from build123d import *

# Parameters (mm, degrees)
F0_W     = 63.351966
F0_H     = 58.721166
F1_DEPTH = 50.8
F2_R     = 6.67715
F3_DEPTH = 25.4
F4_R     = 5.78901
F5_DEPTH = 25.4
F6_R     = 13.653807
F7_DEPTH = 38.1


with BuildPart() as f1:
    # F0 (on Top) → F1 (new body)
    with BuildSketch(Plane.XY):
        with Locations((31.675983, 29.360583)):
            Rectangle(F0_W, F0_H)
    extrude(amount=F1_DEPTH)

    # F2 (on face) → F3 (cut)
    with BuildSketch(Plane.XY.offset(50.8)):
        with Locations((47.149416, 48.132766)):
            Circle(F2_R)
    extrude(amount=-F3_DEPTH, mode=Mode.SUBTRACT)

    # F4 (on face) → F5 (cut)
    with BuildSketch(Plane(origin=(0, 0, 0), x_dir=(1, 0, 0), z_dir=(0, 0, -1))):
        with Locations((9.225111, -8.943532)):
            Circle(F4_R)
    extrude(amount=-F5_DEPTH, mode=Mode.SUBTRACT)

    # F6 (on face) → F7 (cut)
    with BuildSketch(Plane(origin=(0, 0, 0), x_dir=(0, -1, 0), z_dir=(-1, 0, 0))):
        with Locations((0, 50.8)):
            Circle(F6_R)
    extrude(amount=-F7_DEPTH, mode=Mode.SUBTRACT)


solid = f1.part
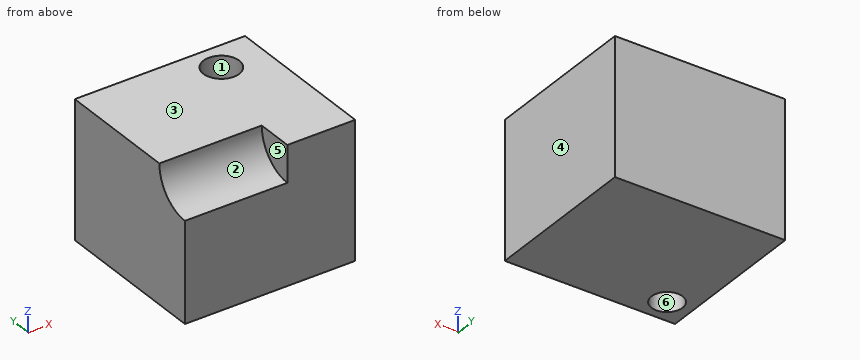
Verification items for the finished model (mm, model axes). Face numbers are marked on the shaded views. A direction names the side the tool comes from. Coordinates: 2 decimals unless noted, no trailing zeros. Order: outer loops, then holes, each group sorted by start corner. A loop starts at its lowest first (then second) coordinate and runs counter-clockwise, first axis right, second up. Notation, with made-up numbers: (13.25, -2) -> (18.25, -2) arc R17 cw to (18.25, 11) -> close; hole circle Ø9 at (66.25, 66). An arc over 180 degrees is marked (long way). Put each result on its own line as item: value. Start each with the question number.
1. Access from +Z, -Z, +X, -X, +Y, -Y to the whole of each face (thin tool, end or side, straight path). Record for the marked faces 4, 5 and 6.
2. Cross-section at B-B, the plane y = 49.5. Record the boundary of the cut face in (x, z), then the cut area to 3 significant figures.
3. Cross-section at D-D, the plane x = 25. Record the boundary of the cut face in (y, z), then the cut area to 3 significant figures.
4. Cross-section at A-A, the plane x = 8. Record the boundary of the cut face in (y, z), then the cut area to 3 significant figures.
5. Material ranges on L1, parallel to X at y = 8.5, z = 21.5; L2, parallel to Z at x = 50, y = 42.5; L3, parallel to Y at x = 49, z = 40.5, recorded low to high. Write a range as [from, to].
6. Go/stop test with flat-tipped pins: pin 1 Ø7 at (y, z) = (4.5, 45) entering from -X; pin 2 Ø10.5 at (x, y) = (47.15, 48.13) entering from +Z. Record where each tip stops, or that it passes through.
7. Mould release check, pull along Y, two halves, no side actions. Record for the marked faces 1, 2 and 3: released by +Y, released by -Y, zero draft, split by the parting line, or undercut.
8. Cross-section at C-C, the plane z = 13.5. Record the boundary of the cut face in (x, y).
Computed:
1. face 4: +Z, -Z, +X, +Y, -Y
1. face 5: +Z, -X, -Y
1. face 6: -Z
2. outline: (0, 0) -> (63.35, 0) -> (63.35, 50.8) -> (53.69, 50.8) -> (53.69, 25.4) -> (40.61, 25.4) -> (40.61, 50.8) -> (0, 50.8) -> close
2. area: 2,890 mm2
3. outline: (0, 0) -> (58.72, 0) -> (58.72, 50.8) -> (13.65, 50.8) arc R13.65 cw to (0, 37.15) -> close
3. area: 2,840 mm2
4. outline: (0, 0) -> (3.29, 0) -> (3.29, 25.4) -> (14.6, 25.4) -> (14.6, 0) -> (58.72, 0) -> (58.72, 50.8) -> (13.65, 50.8) arc R13.65 cw to (0, 37.15) -> close
4. area: 2,550 mm2
5. L1: [0, 3.45], [15, 63.35]
5. L2: [0, 25.4]
5. L3: [0, 41.72], [54.55, 58.72]
6. pin 1: x = 38.1
6. pin 2: z = 25.4
7. face 1: undercut
7. face 2: released by -Y
7. face 3: zero draft
8. outline: (0, 0) -> (63.35, 0) -> (63.35, 58.72) -> (0, 58.72) -> close; hole circle Ø11.58 at (9.23, 8.94)
